from build123d import *

# Parameters (mm, degrees)
CROQUIS1_R              = 55
SALIENTE_EXTRUIR1_DEPTH = 7
CROQUIS2_R              = 51
CORTAR_EXTRUIR1_DEPTH   = 5.5
CORTAR_EXTRUIR2_REACH   = 80.096
CROQUIS3_R              = 19


with BuildPart() as part:
    # Croquis1 → Saliente-Extruir1 (new body)
    with BuildSketch(Plane(origin=(0, 0, 0), x_dir=(1, 0, 0), z_dir=(0, 1, 0))):
        with Locations(Location((0, 0, 0), (0, 0, 270))):
            Circle(CROQUIS1_R)
    extrude(amount=SALIENTE_EXTRUIR1_DEPTH)

    # Croquis2 → Cortar-Extruir1 (cut)
    with BuildSketch(Plane.XZ):
        with Locations(Location((0, 0, 0), (0, 0, 270))):
            Circle(CROQUIS2_R)
    extrude(amount=-CORTAR_EXTRUIR1_DEPTH, mode=Mode.SUBTRACT)

    # Croquis3 → Cortar-Extruir2 (cut, up to next)
    with BuildSketch(Plane(origin=(0, 7, 0), x_dir=(1, 0, 0), z_dir=(0, 1, 0)), mode=Mode.PRIVATE) as cortar_extruir2_sk1:
        with Locations(Location((0, 0, 0), (0, 0, 270))):
            Circle(CROQUIS3_R)
    cortar_extruir2_tool1 = extrude(cortar_extruir2_sk1.sketch, amount=-CORTAR_EXTRUIR2_REACH, mode=Mode.PRIVATE) & part.part
    add(cortar_extruir2_tool1.solids().sort_by_distance((0, 7, 0))[0], mode=Mode.SUBTRACT)


solid = part.part
Build history of the part. All positions in model axes, mm. A direction names the side the tool comes from. Round coordinates to 2 decimals unless told otherwise and drop trailing zeros. Write each loop counter-clockwise with the first axis right and the second up, starting at its lowest first coordinate (ties: lowest second). Pieces come first, ordered by that corner, then holes. Notation, with made-up numbers: M -37.75,-18 L -18.75,-18 A17 ccw -18.75,-9 Z; hole C 9,-33.5 d9. An arc over 180 degrees is marked long. Answer in a Markdown table with one row per item.
1. Saw through at C-C (z = -46). List the corners of the cut face in (x, y).
Geometry check:
| item | result |
|---|---|
| outline | M -30.15,0 L -22.02,0 L -22.02,5.5 L 22.02,5.5 L 22.02,0 L 30.15,0 L 30.15,7 L -30.15,7 Z |
2. Probe L1, parallel to X at y = 6, z = 0; L2, parallel to X at y = 2, z = 0; L3, parallel to Y at x = -29, z = -29.5. List the from-to ranges inside material, lowest first. Write a range as [from, to].
Geometry check:
| item | result |
|---|---|
| L1 | [-55, -19], [19, 55] |
| L2 | [-55, -51], [51, 55] |
| L3 | [5.5, 7] |
3. Saw through at D-D (y = 3.5). List the corners of the cut face in (x, z), and give its area (3 significant figures).
Geometry check:
| item | result |
|---|---|
| outline | C 0,0 d110; hole C 0,0 d102 |
| area | 1,330 mm2 |
4. Mould opens along X. For faces 3 (the face through (-48.794, 3.451, 25.379)), 4 (the face through (-24, 7, -1)), 5 (the face through (1, 5.5, -22)) say: +X half, -X half, draft (parallel to the pull), parting line (faces both ways), or undercut.
Geometry check:
| item | result |
|---|---|
| face 3 | parting line |
| face 4 | draft |
| face 5 | undercut |
5. Saw through at B-B (z = 0). List the corners of the cut face in (x, y).
Geometry check:
| item | result |
|---|---|
| outline | M -55,0 L -51,0 L -51,5.5 L -19,5.5 L -19,7 L -55,7 Z; M 19,5.5 L 51,5.5 L 51,0 L 55,0 L 55,7 L 19,7 Z |
6. Saw through at A-A (x = 0). List the corners of the cut face in (y, z), and give its area (3 significant figures).
Geometry check:
| item | result |
|---|---|
| outline | M 0,-55 L 7,-55 L 7,-19 L 5.5,-19 L 5.5,-51 L 0,-51 Z; M 0,51 L 5.5,51 L 5.5,19 L 7,19 L 7,55 L 0,55 Z |
| area | 152 mm2 |
7. Flat gauge pins, fed straight in: P1, Ø1.5, axis at x = 35.5, y = 2.5, coming from the +Z side; P2, Ø4, axis at x = -29, y = 3, coming from the -Z side; P3, Ø4, axis at y = 6, z = -10.5, coming from the -X side. Where does each tip first touch, or does it go through?
Geometry check:
| item | result |
|---|---|
| P1 | z = 42.63 |
| P2 | z = -47.92 |
| P3 | x = -54.34 |
8. Which spindle directions (+Z, -Z, +X, -X, +Y, -Y) get a long thin tool onto all of the face, cutting with end or side? Do faces 1 (the face through (-49.787, 2.712, 11.056)), 2 (the face through (-16, 0, 49)). Say none if no direction does.
Geometry check:
| item | result |
|---|---|
| face 1 | -Y |
| face 2 | +Z, -Z, +X, -X, -Y |
